Here's how the part is built. I have some questions about the finished solid (model axes, mm). A direction names the side the tool comes from. Give positions to 0.01 mm unless a question says otherwise; leave off trailing zeros. Loops run counter-clockwise (first coordinate to the right, second up) from the corner with the lowest first, then second, coordinate; pieces in that order, holes last. Notation, with made-up numbers: (-21.75, 23) -> (3.25, 23) arc R32 cw to (3.25, 58) -> close; hole circle Ø5 at (78, -27). An arc over 180 degrees is marked (long way). Answer in a Markdown table with one row per item. Add a question column.
Item 1: If we section it at C-C (x = -31): Write out the boundary of the cut face in (y, z) (3 decimals), then the cut area to 3 significant figures.
Item 2: If we section it at D-D (z = -1.5): Write out the boundary of the cut face in (x, y) (3 decimals).
Item 3: We'd pull the mould along Y, two halves only. Please class faces 1 (the face through (-68.5, 4, 3)), 2 (the face through (-62.09, -13.44, 3.04)), 3 (the face through (24.58, 13.14, 1.73)): released by +Y, released by -Y, zero draft, split by the parting line, or undercut.
Item 4: If we section it at B-B (x = 22.5): Write out the boundary of the cut face in (y, z) (3 decimals).
Item 5: Which directions (+Z, -Z, +X, -X, +Y, -Y) give clear straight access to the entire face, cutting with the end or side of a thin tool? Please do faces 4 (the face through (-1, 6.955, -2)), 5 (the face through (-59.36, 4.87, -1.97)), 6 (the face through (59.254, 4.974, -1.972)), 7 (the face through (55.5, -16, 4)), 8 (the face through (-1, 5, 1)).
Item 6: If we section it at A-A (y = 14): Write out the boundary of the cut face in (x, z), then the cut area to 4 significant figures.
Item 7: For P1, Ø7, axis at x = -22.5, y = 14, coming from the +Z side; P2, Ø6, axis at x = -22.5, y = -14, coming from the -Z side; P3, Ø1.2, axis at x = -0.5, z = -2, coming from the -Y side (3 decimals); P4, Ø2.5, axis at x = 22.5, y = 14, coming from the -Z side, each with a flat end and sliding along its axis, tell me the tip position at first contact or that it passes through.
Item 8: If I drill on line 1 (Y direction, x = -22.5, z = 2.45); line 2 (X direction, y = -14, z = 2.4); line 3 (Y direction, x = -47, z = -2) (3 decimals), over which ranges is the centre line in solid material (lowest first)?
```python
from build123d import *

# Parameters (mm, degrees)
F1_DEPTH       = 6
F3_DEPTH       = 13
F5_D           = 4.5
F5_CSINK_D     = 9.5
F5_CSINK_ANGLE = 90
F7_W           = 110
F7_H           = 10
F8_DEPTH       = 4
F9_SIZE        = 3


with BuildPart() as f1:
    # F0 (on Top) → F1 (new body)
    with BuildSketch(Plane.XY):
        Polygon((0, 20), (-68.5, 20), (-68.5, -20), (0, -20), (0, -5), (-55, -5), (-55, 5), (0, 5), align=None)
    extrude(amount=F1_DEPTH)

    # F2 (on face) → F3 (cut)
    with BuildSketch(Plane(origin=(-68.5, 0, 0), x_dir=(0, -1, 0), z_dir=(-1, 0, 0))):
        Polygon((20, 0), (20, 6), (9, 6), (18, 0), align=None)
    extrude(amount=-F3_DEPTH, mode=Mode.SUBTRACT)

    # F5 (through all)
    with Locations(Plane.XY.offset(6)):
        with Locations((-22.5, 14), (-22.5, -14)):
            CounterSinkHole(F5_D / 2, F5_CSINK_D / 2, counter_sink_angle=F5_CSINK_ANGLE)

    # F6: F1 across plane


with BuildPart() as f1_1:
    add(f1.part)
    add(f1.part.mirror(Plane.YZ))

    # F7 (on face) → F8 (join)
    with BuildSketch(Plane(origin=(0, 0, 0), x_dir=(1, 0, 0), z_dir=(0, 0, -1))):
        with BuildLine():
            Line((54.375, 6.955), (-54.375, 6.955))
            ThreePointArc((-54.375, 6.955), (-59.3088119137, 4.9206318833), (-61.3748553556, 0))
            ThreePointArc((-61.3748553556, 0), (-59.3088119137, -4.9206318833), (-54.375, -6.955))
            Line((-54.375, -6.955), (54.375, -6.955))
            ThreePointArc((54.375, -6.955), (59.3088119137, -4.9206318833), (61.3748553556, 0))
            ThreePointArc((61.3748553556, 0), (59.3088119137, 4.9206318833), (54.375, 6.955))
        make_face()
        Rectangle(F7_W, F7_H, mode=Mode.SUBTRACT)
    extrude(amount=F8_DEPTH)

    # F9
    f9_edges = [f1_1.edges().sort_by_distance(p)[0] for p in [
        (-68.5, 20, 3),
        (68.5, 20, 3),
    ]]
    chamfer(f9_edges, length=F9_SIZE)


solid = f1_1.part
```
Recorded:
| question | item | result |
|---|---|---|
| 1 | outline | (-20, 0) -> (-6.955, 0) -> (-6.955, -4) -> (-5, -4) -> (-5, 6) -> (-20, 6) -> close; (5, -4) -> (6.955, -4) -> (6.955, 0) -> (20, 0) -> (20, 6) -> (5, 6) -> close |
| 1 | area | 196 mm^2 |
| 2 | outline | (-61.375, 0) arc R7 ccw to (-54.375, -6.955) -> (54.375, -6.955) arc R7 ccw to (61.375, 0) arc R7 ccw to (54.375, 6.955) -> (-54.375, 6.955) arc R7 ccw to start; hole (-55, -5) -> (55, -5) -> (55, 5) -> (-55, 5) -> close |
| 3 | face 1 | zero draft |
| 3 | face 2 | released by -Y |
| 3 | face 3 | undercut |
| 4 | outline | (-20, 0) -> (-16.25, 0) -> (-16.25, 3.5) -> (-18.75, 6) -> (-20, 6) -> close; (-11.75, 0) -> (-6.955, 0) -> (-6.955, -4) -> (-5, -4) -> (-5, 6) -> (-9.25, 6) -> (-11.75, 3.5) -> close; (5, -4) -> (6.955, -4) -> (6.955, 0) -> (11.75, 0) -> (11.75, 3.5) -> (9.25, 6) -> (5, 6) -> close; (16.25, 0) -> (20, 0) -> (20, 6) -> (18.75, 6) -> (16.25, 3.5) -> close |
| 5 | face 4 | -Z, +X, -X, +Y |
| 5 | face 5 | -Z, -X, +Y |
| 5 | face 6 | -Z, +X, +Y |
| 5 | face 7 | +Z, +X, -Y |
| 5 | face 8 | +Z, -Z |
| 6 | outline | (-68.5, 0) -> (-24.75, 0) -> (-24.75, 3.5) -> (-27.25, 6) -> (-68.5, 6) -> close; (-20.25, 0) -> (20.25, 0) -> (20.25, 3.5) -> (17.75, 6) -> (-17.75, 6) -> (-20.25, 3.5) -> close; (24.75, 0) -> (68.5, 0) -> (68.5, 6) -> (27.25, 6) -> (24.75, 3.5) -> close |
| 6 | area | 755.5 mm^2 |
| 7 | P1 | stops at z = 4.75 |
| 7 | P2 | stops at z = 0 |
| 7 | P3 | stops at y = -6.955 |
| 7 | P4 | passes through |
| 8 | line 1 | y = -20 to -16.25, -11.75 to -5, 5 to 11.75, 16.25 to 20 |
| 8 | line 2 | x = -68.5 to -24.75, -20.25 to 20.25, 24.75 to 68.5 |
| 8 | line 3 | y = -6.955 to -5, 5 to 6.955 |
